from build123d import *

# Parameters (mm, degrees)
SKETCH1_W                                      = 35
SKETCH1_H                                      = 6
BOSS_EXTRUDE1_DEPTH                            = 76
SKETCH2_R                                      = 1.6
CUT_EXTRUDE1_DEPTH                             = 84.886828525
SKETCH3_R                                      = 1
CUT_EXTRUDE2_DEPTH                             = 4
CBORE_START                                    = -6
CBORE_SLOT_FOR_M3_HEX_SOCKET_HEAD_CAP_SC_DEPTH = 3.4
CBORE_START_2                                  = -2.6
CBORE_SLOT_FOR_M3_HEX_SOCKET_HEAD_CA_3_DEPTH   = 2.6
CUT_EXTRUDE3_DEPTH                             = 84.886828525
SKETCH8_R                                      = 1.25
CUT_EXTRUDE4_DEPTH                             = 84.886828525


# Read off the part's stored shape, not the designer's step: CBORE SLOT for M3 Hex Socket Head Cap Screw1
with BuildPart() as part:
    # Sketch1 → Boss-Extrude1 (new body)
    with BuildSketch(Plane(origin=(0, 0, 0), x_dir=(1, 0, 0), z_dir=(0, 1, 0))):
        with Locations((17.5, 3)):
            Rectangle(SKETCH1_W, SKETCH1_H)
    extrude(amount=BOSS_EXTRUDE1_DEPTH)

    # Sketch2 → Cut-Extrude1 (cut, through all)
    with BuildSketch(Plane.XY):
        with Locations((4.5, 73.5)):
            Circle(SKETCH2_R)
        with Locations((30.5, 73.5)):
            Circle(SKETCH2_R)
    extrude(amount=-CUT_EXTRUDE1_DEPTH, mode=Mode.SUBTRACT)

    # Sketch3 → Cut-Extrude2 (cut)
    with BuildSketch(Plane.XY):
        with Locations((10.5, 73.5)):
            Circle(SKETCH3_R)
        with Locations((24.5, 73.5)):
            Circle(SKETCH3_R)
    extrude(amount=-CUT_EXTRUDE2_DEPTH, mode=Mode.SUBTRACT)

    # CBORE SLOT for M3 Hex Socket Head Ca 2 → CBORE SLOT for M3 Hex Socket Head Cap Screw1 (cut)
    with BuildSketch(Plane.XY.offset(CBORE_START)):
        with BuildLine():
            ThreePointArc((8.25, 46.4), (5, 49.65), (1.75, 46.4))
            Line((1.75, 46.4), (1.75, 42.6))
            ThreePointArc((1.75, 42.6), (5, 39.35), (8.25, 42.6))
            Line((8.25, 42.6), (8.25, 46.4))
        make_face()
        with BuildLine():
            ThreePointArc((33.25, 46.4), (30, 49.65), (26.75, 46.4))
            Line((26.75, 46.4), (26.75, 42.6))
            ThreePointArc((26.75, 42.6), (30, 39.35), (33.25, 42.6))
            Line((33.25, 42.6), (33.25, 46.4))
        make_face()
    extrude(amount=CBORE_SLOT_FOR_M3_HEX_SOCKET_HEAD_CAP_SC_DEPTH, mode=Mode.SUBTRACT)

    # CBORE SLOT for M3 Hex Socket Head Ca 3 o → CBORE SLOT for M3 Hex Socket Head Ca 3 (cut)
    with BuildSketch(Plane.XY.offset(CBORE_START_2)):
        with BuildLine():
            ThreePointArc((6.6, 46.4), (5, 48), (3.4, 46.4))
            Line((3.4, 46.4), (3.4, 42.6))
            ThreePointArc((3.4, 42.6), (5, 41), (6.6, 42.6))
            Line((6.6, 42.6), (6.6, 46.4))
        make_face()
        with BuildLine():
            ThreePointArc((31.6, 46.4), (30, 48), (28.4, 46.4))
            Line((28.4, 46.4), (28.4, 42.6))
            ThreePointArc((28.4, 42.6), (30, 41), (31.6, 42.6))
            Line((31.6, 42.6), (31.6, 46.4))
        make_face()
    extrude(amount=CBORE_SLOT_FOR_M3_HEX_SOCKET_HEAD_CA_3_DEPTH, mode=Mode.SUBTRACT)

    # Sketch7 → Cut-Extrude3 (cut, through all)
    with BuildSketch(Plane(origin=(0, 0, -6), x_dir=(-1, 0, 0), z_dir=(0, 0, -1))):
        with BuildLine():
            Line((0, 0), (-19, 0))
            Line((-19, 0), (-19, 34))
            ThreePointArc((-19, 34), (-17.828427125, 36.828427125), (-15, 38))
            Line((-15, 38), (0, 38))
            Line((0, 38), (0, 0))
        make_face()
    extrude(amount=-CUT_EXTRUDE3_DEPTH, mode=Mode.SUBTRACT)

    # Sketch8 → Cut-Extrude4 (cut, through all)
    with BuildSketch(Plane(origin=(0, 0, -6), x_dir=(-1, 0, 0), z_dir=(0, 0, -1))):
        with Locations((-31, 7.5)):
            Circle(SKETCH8_R)
        with Locations(Location((-31, 29.5, 0), (0, 0, 180))):
            Circle(SKETCH8_R)
    extrude(amount=-CUT_EXTRUDE4_DEPTH, mode=Mode.SUBTRACT)


solid = part.part
The model under review builds one solid part; all positions refer to its coordinate system, in mm. A direction names the side the tool comes from. Coordinates: 2 decimals unless noted, no trailing zeros. Loops run counter-clockwise (first coordinate to the right, second up) from the corner with the lowest first, then second, coordinate; pieces in that order, holes last.
(1) Consider section D-D, the plane x = 4.5. Give the boundary of the cut face in (y, z), plus the area to 3 significant figures.
Determined:
outline: (38, -6) - (39.39, -6) - (39.39, -2.6) - (41.08, -2.6) - (41.08, 0) - (38, 0) - close; (47.92, -2.6) - (49.61, -2.6) - (49.61, -6) - (71.9, -6) - (71.9, 0) - (47.92, 0) - close; (75.1, -6) - (76, -6) - (76, 0) - (75.1, 0) - close
area: 156 mm2
(2) Insertion check: P1, Ø1, axis at y = 25.5, z = -5, coming from the -X side; P2, Ø0.6, axis at x = 24, y = 73.5, coming from the +Z side. Each pin has a flat end and moves straight along its axis. Give the tip position at first contact, or say it passes through.
Determined:
P1: stops at x = 19
P2: stops at z = -4
(3) Wall thickness on L1, parallel to X at y = 73.5, z = -4.25; L2, parallel to X at y = 73.5, z = -1.9; L3, parallel to Y at x = 24.5, z = -1.2: over which ranges is each line inside the solid? List them lowest first.
Determined:
L1: x = 0 to 2.9, 6.1 to 28.9, 32.1 to 35
L2: x = 0 to 2.9, 6.1 to 9.5, 11.5 to 23.5, 25.5 to 28.9, 32.1 to 35
L3: y = 0 to 72.5, 74.5 to 76
(4) Consider section A-A, the plane y = 73.5. Give the boundary of the cut face in (x, z), plus the area to 3 significant figures.
Determined:
outline: (0, -6) - (2.9, -6) - (2.9, 0) - (0, 0) - close; (6.1, -6) - (28.9, -6) - (28.9, 0) - (25.5, 0) - (25.5, -4) - (23.5, -4) - (23.5, 0) - (11.5, 0) - (11.5, -4) - (9.5, -4) - (9.5, 0) - (6.1, 0) - close; (32.1, -6) - (35, -6) - (35, 0) - (32.1, 0) - close
area: 156 mm2
(5) Tool access review of faces 1 (the cylindrical face through (5, 48, -1)), 2 (the cylindrical face through (30.07, 49.65, -4.32)), 3 (the cylindrical face through (24.96, 72.61, -1.97)): name each direction out of +Z, -Z, +X, -X, +Y, -Y from which nothing blocks a thin tool from reaching the whole face with its end or side.
Determined:
face 1: +Z, -Z
face 2: -Z
face 3: +Z
(6) Draft analysis for pull direction Y (two halves, no side actions). For faces 4 (the flat face through (21, 46, 0)), 5 (the flat face through (17, 76, -3)), 6 (the cylindrical face through (5, 41, -1)), state which applies: +Y half, -Y half, draft (parallel to the pull), parting line (faces both ways), or undercut.
Determined:
face 4: draft
face 5: +Y half
face 6: undercut
(7) Consider section B-B, the plane x = 10.5. Give the boundary of the cut face in (y, z), plus the area to 3 significant figures.
Determined:
outline: (38, -6) - (76, -6) - (76, 0) - (74.5, 0) - (74.5, -4) - (72.5, -4) - (72.5, 0) - (38, 0) - close
area: 220 mm2
(8) Consider section C-C, the plane z = -1.6. Give the number of separate pieces and of enclosed holes in the cut face, plus the area to 3 significant figures.
Determined:
separate pieces: 1
enclosed holes: 8
area: 1,870 mm2
